Check sheet for the modelled part. Datum: model origin and axes. Units: mm. Coordinates: 2 decimals unless noted, no trailing zeros. Loops run counter-clockwise (first coordinate to the right, second up) from the corner with the lowest first, then second, coordinate; pieces in that order, holes last. Notation, with made-up numbers: (84, 1) -> (90, 1) arc R13 cw to (90, 13) -> close; hole circle Ø2 at (50, 48). An arc over 180 degrees is marked (long way). Use CSV: the item, a comma, the result in double quotes.
```python
from build123d import *

# Parameters (mm, degrees)
SKETCH_1_W              = 340.4
SKETCH_1_H              = 900
EXTRUDE_1_DEPTH         = 50
HOLE_WIZARD_M6_3_D      = 5
HOLE_WIZARD_M6_3_DEPTH  = 20
HOLE_WIZARD_M6_3_TIP    = 1.502151548
CUT_EXTRUDE_1_DEPTH     = 1
HOLE_WIZARD_M6_4_D      = 5
HOLE_WIZARD_M6_4_DEPTH  = 15
HOLE_WIZARD_M6_4_TIP    = 1.502151548
HOLE_WIZARD_M6_9_D      = 5
HOLE_WIZARD_M6_9_DEPTH  = 12
HOLE_WIZARD_M6_9_TIP    = 1.502151548
SKETCH_32_W             = 50
SKETCH_32_H             = 900
EXTRUDE_2_DEPTH         = 50
HOLE_WIZARD_M8_2_D      = 6.8
HOLE_WIZARD_M8_2_DEPTH  = 19.75
HOLE_WIZARD_M8_2_TIP    = 2.042926105
FILLET_1_R              = 20
HOLE_WIZARD_M6_12_D     = 5
HOLE_WIZARD_M6_12_DEPTH = 15
HOLE_WIZARD_M6_12_TIP   = 1.502151548
M5_C_1_D                = 5.3
M5_C_1_DEPTH            = 5.2
M5_C_1_CBORE_D          = 11
M5_C_1_CBORE_DEPTH      = 0.5
M5_C_1_TIP              = 1.59228064


with BuildPart() as part:
    # Sketch 1 → Extrude 1 (new body)
    with BuildSketch(Plane(origin=(0, 0, 0), x_dir=(1, 0, 0), z_dir=(0, 1, 0))):
        Rectangle(SKETCH_1_W, SKETCH_1_H)
    extrude(amount=EXTRUDE_1_DEPTH)

    # Hole Wizard M6 _3
    with Locations(Plane(origin=(0, 50, 0), x_dir=(1, 0, 0), z_dir=(0, 1, 0))):
        with Locations((15, 225.980762114), (15, 174.019237886), (-15, 174.019237886), (-30, 200), (-15, 225.980762114), (30, 200)):
            Hole(HOLE_WIZARD_M6_3_D / 2, depth=HOLE_WIZARD_M6_3_DEPTH)
            with Locations((0, 0, -(HOLE_WIZARD_M6_3_DEPTH + HOLE_WIZARD_M6_3_TIP / 2))):  # 118° drill point
                Cone(0, HOLE_WIZARD_M6_3_D / 2, HOLE_WIZARD_M6_3_TIP, mode=Mode.SUBTRACT)

    # Sketch 16 → Cut-Extrude 1 (cut)
    with BuildSketch(Plane(origin=(0, 50, 0), x_dir=(1, 0, 0), z_dir=(0, 1, 0))):
        Polygon((0, -440), (200, -440), (200, -190), (-200, -190), (-200, -440), align=None)
    extrude(amount=-CUT_EXTRUDE_1_DEPTH, mode=Mode.SUBTRACT)

    # Hole Wizard M6 _4
    with Locations(Plane.XZ):
        with Locations((0, 0), (105, 65), (-105, -65), (-105, 65), (105, -65)):
            Hole(HOLE_WIZARD_M6_4_D / 2, depth=HOLE_WIZARD_M6_4_DEPTH)
            with Locations((0, 0, -(HOLE_WIZARD_M6_4_DEPTH + HOLE_WIZARD_M6_4_TIP / 2))):  # 118° drill point
                Cone(0, HOLE_WIZARD_M6_4_D / 2, HOLE_WIZARD_M6_4_TIP, mode=Mode.SUBTRACT)

    # Hole Wizard M6 _9
    with Locations(Plane(origin=(0, 0, 0), x_dir=(-1, 0, 0), z_dir=(0, -1, 0))):
        with Locations((-63, -317.154485024), (63, -317.154485024), (63, -363.154485024), (-63, -363.154485024)):
            Hole(HOLE_WIZARD_M6_9_D / 2, depth=HOLE_WIZARD_M6_9_DEPTH)
            with Locations((0, 0, -(HOLE_WIZARD_M6_9_DEPTH + HOLE_WIZARD_M6_9_TIP / 2))):  # 118° drill point
                Cone(0, HOLE_WIZARD_M6_9_D / 2, HOLE_WIZARD_M6_9_TIP, mode=Mode.SUBTRACT)

    # Sketch 32 → Extrude 2 (add)
    with BuildSketch(Plane.XZ):
        with Locations((-195.2, 0)):
            Rectangle(SKETCH_32_W, SKETCH_32_H)
        with Locations((195.2, 0)):
            Rectangle(SKETCH_32_W, SKETCH_32_H)
    extrude(amount=-EXTRUDE_2_DEPTH)

    # Hole Wizard M8 _2
    with Locations(Plane(origin=(0, 0, 0), x_dir=(-1, 0, 0), z_dir=(0, -1, 0))):
        with Locations((-145, -304.975259132), (-145, -374.975259132), (145, -304.975259132), (145, -374.975259132)):
            Hole(HOLE_WIZARD_M8_2_D / 2, depth=HOLE_WIZARD_M8_2_DEPTH)
            with Locations((0, 0, -(HOLE_WIZARD_M8_2_DEPTH + HOLE_WIZARD_M8_2_TIP / 2))):  # 118° drill point
                Cone(0, HOLE_WIZARD_M8_2_D / 2, HOLE_WIZARD_M8_2_TIP, mode=Mode.SUBTRACT)

    # Fillet 1
    fillet_1_edges = [part.edges().sort_by_distance(p)[0] for p in [
        (-220.2, 25, -450),
        (-220.2, 25, 450),
        (220.2, 25, 450),
        (220.2, 25, -450),
    ]]
    fillet(fillet_1_edges, radius=FILLET_1_R)

    # Hole Wizard M6 _12
    with Locations(Plane(origin=(0, 50, 0), x_dir=(1, 0, 0), z_dir=(0, 1, 0))):
        with Locations((-89.854599393, 405.43620182), (-89.854599393, 345.43620182), (90.145400607, 345.43620182), (90.145400607, 405.43620182)):
            Hole(HOLE_WIZARD_M6_12_D / 2, depth=HOLE_WIZARD_M6_12_DEPTH)
            with Locations((0, 0, -(HOLE_WIZARD_M6_12_DEPTH + HOLE_WIZARD_M6_12_TIP / 2))):  # 118° drill point
                Cone(0, HOLE_WIZARD_M6_12_D / 2, HOLE_WIZARD_M6_12_TIP, mode=Mode.SUBTRACT)

    # M5 _C_1
    with Locations(Plane(origin=(0, 0, 0), x_dir=(-1, 0, 0), z_dir=(0, -1, 0))):
        with Locations((-37.5, 221.64), (37.5, 221.64), (-37.5, 136.64), (37.5, 136.64)):
            CounterBoreHole(M5_C_1_D / 2, M5_C_1_CBORE_D / 2, M5_C_1_CBORE_DEPTH, depth=M5_C_1_DEPTH)
            with Locations((0, 0, -(M5_C_1_DEPTH + M5_C_1_TIP / 2))):  # 118° drill point
                Cone(0, M5_C_1_D / 2, M5_C_1_TIP, mode=Mode.SUBTRACT)


solid = part.part
```
1) Thickness scan on line 1 along X through (y, z) = (0.2, -221.64); line 2 along Z through (x, y) = (-37.5, 0.2); line 3 along Z through (x, y) = (63, 7.25). Record the ranges inside material, lowest first. Write a range as from..to.
Answer below:
line 1,"x = -220.2..-43, -32..32, 43..220.2"
line 2,"z = -450..-227.14, -216.14..-142.14, -131.14..450"
line 3,"z = -450..314.65, 319.65..360.65, 365.65..450"
2) Go/stop test with flat-tipped pins: pin 1 Ø3 at (x, z) = (-105, -65) entering from -Y; pin 2 Ø3 at (x, z) = (90.15, -405.44) entering from +Y; pin 3 Ø4 at (x, z) = (145, 374.98) entering from -Y. Record where each tip stops, or that it passes through.
Answer below:
pin 1,"stops at y = 15.6"
pin 2,"stops at y = 34.4"
pin 3,"stops at y = 20.59"
3) Draft check along Z on faces 1 (the cylindrical face through (214.186, 25.35, 444.297)), 2 (the flat face through (-2, 49, 313)), 3 (the cylindrical face through (214.186, 25.35, -444.297)). Enter one of: released by +Z, released by -Z, zero draft, split by the parting line, or undercut.
Answer below:
face 1,"released by +Z"
face 2,"undercut"
face 3,"released by -Z"
4) Cross-section at A-A on z = 246. Record the boundary of the cut face in (x, y), and give its area (3 significant figures).
Answer below:
outline,"(-220.2, 0) -> (220.2, 0) -> (220.2, 50) -> (170.2, 50) -> (170.2, 49) -> (-170.2, 49) -> (-170.2, 50) -> (-220.2, 50) -> close"
area,"21,700 mm²"
